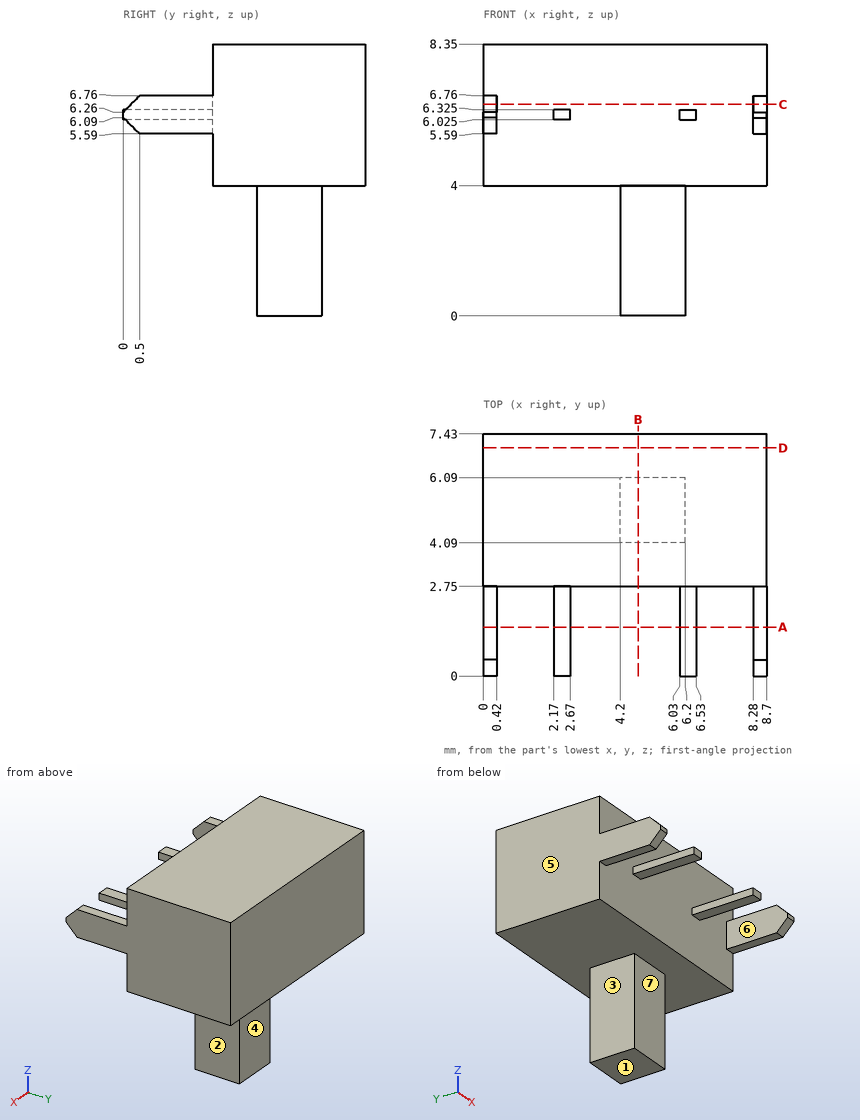
Geometry check sheet. Reference: drawing and pictorial views, mm from the part's lowest x, y, z. A direction names the side the tool comes from. Give positions to 0.01 mm unless a question says otherwise; leave off trailing zeros. Order: outer loops, then holes, each group sorted by start corner. A loop starts at its lowest first (then second) coordinate and runs counter-clockwise, first axis right, second up. Notation, with made-up numbers: M 64,16 L 84,16 A27 ccw 84,47 Z; hole C 80,57 d10. An arc over 180 degrees is marked long. Answer in a Markdown table with one row per item. Add a question column.
Q1. Sectioned sample at B-B, the plane x = 4.75. Record the boundary of the cut face in (y, z).
Q2. Sectioned sample at D-D, the plane y = 7. Record the boundary of the cut face in (x, z), and give its area (3 significant figures).
Q3. Gauge pin test, flat ends, axial feed: pin 1 Ø1.6 at (y, z) = (5, 1.5) entering from +X; pin 2 Ø0.5 at (x, y) = (0.5, 1.5) entering from -Z; pin 3 Ø0.6 at (x, z) = (5, 3) entering from +Y; pin 4 Ø1.5 at (y, z) = (1.5, 1) entering from -X. Record the tip position at first contact, or that the pin passes through.
Q4. Sectioned sample at A-A, the plane y = 1.5. Record the boundary of the cut face in (x, z) (3 decimals), and give its area (3 significant figures).
Q5. Release check for a two-part mould opening along X. For the marked faces 5, 6 and 7 record: released by +X, released by -X, zero draft, split by the parting line, or undercut.
Q6. Sectioned sample at C-C, the plane z = 6.5. Record the boundary of the cut face in (x, y), and give its area (3 significant figures).
Q7. Access from +Z, -Z, +X, -X, +Y, -Y to the whole of each face (thin tool, end or side, straight path). Record for the marked faces 1, 2, 3 and 4.
Q8. Thickness scan on L1, parallel to Y at x = 5.5, z = 0.75; L2, parallel to Z at x = 3.75, y = 6.75; L3, parallel to Y at x = 5.5, z = 7. Record the ranges inside material, lowest first.
Verdict:
| question | item | result |
|---|---|---|
| 1 | outline | M 2.75,4 L 4.09,4 L 4.09,0 L 6.09,0 L 6.09,4 L 7.43,4 L 7.43,8.35 L 2.75,8.35 Z |
| 2 | outline | M 0,4 L 8.7,4 L 8.7,8.35 L 0,8.35 Z |
| 2 | area | 37.8 mm² |
| 3 | pin 1 | x = 6.2 |
| 3 | pin 2 | z = 5.59 |
| 3 | pin 3 | y = 6.09 |
| 3 | pin 4 | through |
| 4 | outline | M 0,5.59 L 0.42,5.59 L 0.42,6.76 L 0,6.76 Z; M 2.17,6.025 L 2.67,6.025 L 2.67,6.325 L 2.17,6.325 Z; M 6.03,6.025 L 6.53,6.025 L 6.53,6.325 L 6.03,6.325 Z; M 8.28,5.59 L 8.7,5.59 L 8.7,6.76 L 8.28,6.76 Z |
| 4 | area | 1.28 mm² |
| 5 | face 5 | released by -X |
| 5 | face 6 | undercut |
| 5 | face 7 | zero draft |
| 6 | outline | M 0,0.24 L 0.42,0.24 L 0.42,2.75 L 8.28,2.75 L 8.28,0.24 L 8.7,0.24 L 8.7,7.43 L 0,7.43 Z |
| 6 | area | 42.8 mm² |
| 7 | face 1 | -Z, +X, -X, +Y, -Y |
| 7 | face 2 | -Z, +X, +Y, -Y |
| 7 | face 3 | -Z, -X, +Y, -Y |
| 7 | face 4 | -Z, +X, -X, +Y |
| 8 | L1 | 4.09 to 6.09 |
| 8 | L2 | 4 to 8.35 |
| 8 | L3 | 2.75 to 7.43 |
